For this review, take the finished solid that the model builds, in its own axes (mm). Face numbers are marked on the shaded views. A direction names the side the tool comes from. Give positions to 0.01 mm unless a question says otherwise; leave off trailing zeros. Order: outer loops, then holes, each group sorted by start corner. A loop starts at its lowest first (then second) coordinate and runs counter-clockwise, first axis right, second up. Notation, with made-up numbers: (48.25, 6.5) -> (69.25, 6.5) arc R11 ccw to (69.25, 12.5) -> close; hole circle Ø3 at (79, -8). An arc over 180 degrees is marked (long way). Return JSON: item names as keys, results as strings. Group by question number.
1) Add section B-B (z = 3.75). Give the boundary of the cut face in (x, y).
2) For the marked faces 5, 6 and 7, list the 3-axis set-ups (+Z, -Z, +X, -X, +Y, -Y) from which the entire face can be reached by the end or side of a thin tool; tool diameter is ignored.
3) Add section A-A (x = -0.6). Give the boundary of the cut face in (y, z) (3 decimals).
4) The part is to be moulded in two halves that separate along Y. For the marked faces 1, 2, 3 and 4, say which applies: released by +Y, released by -Y, zero draft, split by the parting line, or undercut.
5) Add section D-D (x = 0.4). Give the boundary of the cut face in (y, z) (3 decimals), then the cut area to 3 significant figures.
6) To check wall thickness, follow line 1 along Y through (x, z) = (-0.15, 2.15); line 2 along Y through (x, z) = (0.1, 2.8); line 3 along Z through (x, y) = (0.25, 5.25) (3 decimals). State the ranges of each line that lie inside material, in increasing order.
7) Insertion check: P1, Ø0.6, axis at x = -0.5, z = 3.5, coming from the +Y side. The pin has a flat end and moves straight along its axis. Give the tip position at first contact, or say it passes through.
8) Add section C-C (z = 2). Give the boundary of the cut face in (x, y), then the cut area to 3 significant figures.
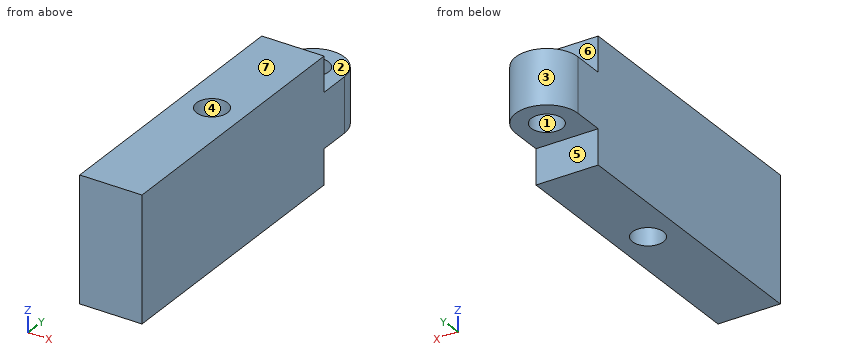
from build123d import *

# Parameters (mm, degrees)
SKETCH_1_R               = 0.5
EXTRUDE_1_DEPTH          = 4
CUT_EXTRUDE_2_DEPTH      = 8.679442038
CUT_EXTRUDE_2_DEPTH_BACK = 8.679442038
SKETCH_2_W               = 1.125
SKETCH_2_H               = 2


with BuildPart() as part:
    # 草图1 → 凸台-拉伸1 (new body)
    with BuildSketch(Plane.XY):
        with BuildLine():
            Line((-1.244261308, -4.563724383), (-1.244261308, 5.436275617))
            ThreePointArc((-1.244261308, 5.436275617), (-0.244261308, 6.436275617), (0.755738692, 5.436275617))
            Line((0.755738692, 5.436275617), (0.755738692, -4.563724383))
            Line((0.755738692, -4.563724383), (-1.244261308, -4.563724383))
        make_face()
        with Locations((-0.244261308, 5.436275617)):
            Circle(SKETCH_1_R, mode=Mode.SUBTRACT)
        with Locations((-0.244261308, 0.436275617)):
            Circle(SKETCH_1_R, mode=Mode.SUBTRACT)
    extrude(amount=EXTRUDE_1_DEPTH)

    # 草图2 → 切除-拉伸2 (cut, two sides: drawn at the far end of the back side and taken through both)
    with BuildSketch(Plane(origin=(0, 0, 0), x_dir=(0, 0, -1), z_dir=(1, 0, 0)).offset(-CUT_EXTRUDE_2_DEPTH_BACK)):
        with Locations((-3.4375, 5.436275617)):
            Rectangle(SKETCH_2_W, SKETCH_2_H)
        with Locations((-0.5625, 5.436275617)):
            Rectangle(SKETCH_2_W, SKETCH_2_H)
    extrude(amount=CUT_EXTRUDE_2_DEPTH + CUT_EXTRUDE_2_DEPTH_BACK, mode=Mode.SUBTRACT)


solid = part.part
Evaluation:
{
 "1": {"outline": "(-1.24, -4.56) -> (0.76, -4.56) -> (0.76, 4.44) -> (-1.24, 4.44) -> close; hole circle Ø1 at (-0.24, 0.44)"},
 "2": {"face 5": "-Z, +X, -X, +Y", "face 6": "+Z, +X, -X, +Y", "face 7": "+Z, +X, -X, +Y, -Y"},
 "3": {"outline": "(-4.564, 0) -> (0.085, 0) -> (0.085, 4) -> (-4.564, 4) -> close; (0.788, 0) -> (4.436, 0) -> (4.436, 1.125) -> (5.085, 1.125) -> (5.085, 2.875) -> (4.436, 2.875) -> (4.436, 4) -> (0.788, 4) -> close; (5.788, 1.125) -> (6.371, 1.125) -> (6.371, 2.875) -> (5.788, 2.875) -> close"},
 "4": {"face 1": "undercut", "face 2": "zero draft", "face 3": "released by +Y", "face 4": "undercut"},
 "5": {"outline": "(-4.564, 0) -> (4.436, 0) -> (4.436, 1.125) -> (6.201, 1.125) -> (6.201, 2.875) -> (4.436, 2.875) -> (4.436, 4) -> (-4.564, 4) -> close", "area": "39.1 mm^2"},
 "6": {"line 1": "-4.56 to -0.05, 0.93 to 4.95, 5.93 to 6.43", "line 2": "-4.56 to 0.07, 0.8 to 5.07, 5.8 to 6.38", "line 3": "1.125 to 2.875"},
 "7": {"P1": "y = 4.44"},
 "8": {"outline": "(-1.24, -4.56) -> (0.76, -4.56) -> (0.76, 5.44) arc R1 ccw to (-1.24, 5.44) -> close; hole circle Ø1 at (-0.24, 0.44); hole circle Ø1 at (-0.24, 5.44)", "area": "20.0 mm^2"}
}
